from build123d import *

# Parameters (mm, degrees)
BOSS_EXTRUDE1_DEPTH = 5
SKETCH2_R           = 4
CUT_EXTRUDE1_DEPTH  = 152.449757015
FILLET1_R           = 6
FILLET2_R           = 3


with BuildPart() as part:
    # Sketch1 → Boss-Extrude1 (new body)
    with BuildSketch(Plane.XY):
        with BuildLine():
            Line((0, 0), (130.17, 0))
            Line((130.17, 0), (150.17, 0))
            Line((150.17, 0), (150.17, -4))
            Line((150.17, -4), (150.17, -12.5))
            ThreePointArc((150.17, -12.5), (143.67, -19), (137.17, -12.5))
            Line((137.17, -12.5), (137.17, -4))
            Line((137.17, -4), (13, -4))
            Line((13, -4), (13, -12.5))
            ThreePointArc((13, -12.5), (6.5, -19), (0, -12.5))
            Line((0, -12.5), (0, -4))
            Line((0, -4), (0, 0))
        make_face()
    extrude(amount=BOSS_EXTRUDE1_DEPTH)

    # Sketch2 → Cut-Extrude1 (cut, through all)
    with BuildSketch(Plane.XY.offset(5)):
        with Locations((6.5, -12.5)):
            Circle(SKETCH2_R)
        with Locations((143.67, -12.5)):
            Circle(SKETCH2_R)
    extrude(amount=-CUT_EXTRUDE1_DEPTH, mode=Mode.SUBTRACT)

    # Fillet1
    fillet1_edges = [part.edges().sort_by_distance(p)[0] for p in [
        (0, 0, 2.5),
        (150.17, 0, 2.5),
    ]]
    fillet(fillet1_edges, radius=FILLET1_R)

    # Fillet2
    fillet2_edges = [part.edges().sort_by_distance(p)[0] for p in [
        (137.17, -4, 2.5),
        (13, -4, 2.5),
    ]]
    fillet(fillet2_edges, radius=FILLET2_R)


solid = part.part
Geometry: final body of the model. Coordinates: model frame, mm. A direction names the side the tool comes from. Round coordinates to 2 decimals unless told otherwise and drop trailing zeros. Loops run counter-clockwise (first coordinate to the right, second up) from the corner with the lowest first, then second, coordinate; pieces in that order, holes last. Notation, with made-up numbers: (-10, 41.5) -> (2, 41.5) arc R21 ccw to (2, 78.5) -> close; hole circle Ø1 at (59.25, 75.5). An arc over 180 degrees is marked (long way). One line per question, with ' | ' between items. Start each with the question number.
1. Set-up query: faces 1 (the face through (0, -9, 2)), 2 (the face through (137.17, -10, 2)). Return all of +Z, -Z, +X, -X, +Y, -Y with unobstructed straight access to the full face (end or side cutting, diameter ignored); none if empty.
2. Section B-B on x = 28. Output: boundary loops of the cut face in (y, z), and give its area (3 significant figures).
3. Section A-A on z = 0.8. Output: boundary loops of the cut face in (x, y), and give its area (3 significant figures).
4. Contact query for a flat-ended pin moving along its axis: pin 1 (2.5 mm diameter, centred on x = 53.5, z = 1.5, fed in from -Y). Output: stop coordinate, or through.
5. Line query: line 1 along Y through (x, z) = (6.5, 2.3); line 2 along X through (y, z) = (-12.75, 0.6); line 3 along X through (y, z) = (-9, 4.15). Output: solid intervals per line, ascending. Write a range as [from, to].
6. Mould query, pull axis X, two halves, no side actions, for faces 3 (the face through (76, -4, 2)), 4 (the face through (13, -10, 2)), 5 (the face through (150.17, -9, 2)), 6 (the face through (75, -3, 0)). Classes: pulls with the +X half, pulls with the -X half, needs draft (parallel to the pull), parting line crosses it, or undercut.
Returned:
1) face 1: +Z, -Z, -X, +Y, -Y | face 2: +Z, -Z, -Y
2) outline: (-4, 0) -> (0, 0) -> (0, 5) -> (-4, 5) -> close | area: 20.0 mm2
3) outline: (0, -12.5) arc R6.5 ccw to (13, -12.5) -> (13, -7) arc R3 cw to (16, -4) -> (134.17, -4) arc R3 cw to (137.17, -7) -> (137.17, -12.5) arc R6.5 ccw to (150.17, -12.5) -> (150.17, -6) arc R6 ccw to (144.17, 0) -> (6, 0) arc R6 ccw to (0, -6) -> close; hole circle Ø8 at (6.5, -12.5); hole circle Ø8 at (143.67, -12.5) | area: 842 mm2
4) pin 1: stops at y = -4
5) line 1: y = [-19, -16.5], [-8.5, 0] | line 2: x = [0, 2.51], [10.49, 13], [137.17, 139.68], [147.66, 150.17] | line 3: x = [0, 4.56], [8.44, 13], [137.17, 141.73], [145.61, 150.17]
6) face 3: undercut | face 4: undercut | face 5: pulls with the +X half | face 6: needs draft
